CAD build for the part. Positions are in the model's coordinates, mm. A direction names the side the tool comes from. Round coordinates to 2 decimals unless told otherwise and drop trailing zeros. Write each loop counter-clockwise with the first axis right and the second up, starting at its lowest first coordinate (ties: lowest second). Pieces come first, ordered by that corner, then holes. Notation, with made-up numbers: (-4.5, 54.25) - (43.5, 54.25) arc R16 ccw to (43.5, 62.25) - close; hole circle Ø7 at (55.25, -33). An arc over 180 degrees is marked (long way). Answer in a Markdown table with one row per item.
Autodesk Inventor part; units mm, degrees
ref_plane "YZ Plane" through (0, 0, 0) normal (1, 0, 0) x (0, 1, 0)
ref_plane "XZ Plane" through (0, 0, 0) normal (0, 1, 0) x (-1, 0, 0)
ref_plane "XY Plane" through (0, 0, 0) normal (0, 0, 1) x (1, 0, 0)
sketch "Sketch1" plane through (0, 0, 0) normal (1, 0, 0) x (0, 1, 0)
  line L0 (-1.25, 6.25) -> (1.25, 6.25)
  arc A0 (1.25, -6.25) -> (1.25, 6.25) centre (1.25, 0) ccw
  line L1 (1.25, -6.25) -> (-1.25, -6.25)
  arc A1 (-1.25, 6.25) -> (-1.25, -6.25) centre (-1.25, 0) ccw
  circle A2 centre (0, -10) radius 1.6
  circle A3 centre (0, 10) radius 1.6
  circle A4 centre (8.25, 44.75) radius 1.6
  circle A5 centre (8.25, 65.25) radius 1.6
  line L2 (-1.25, 91.25) -> (1.25, 91.25)
  arc A6 (1.25, 78.75) -> (1.25, 91.25) centre (1.25, 85) ccw
  line L3 (1.25, 78.75) -> (-1.25, 78.75)
  arc A7 (-1.25, 91.25) -> (-1.25, 78.75) centre (-1.25, 85) ccw
  circle A8 centre (0, 75) radius 1.6
  circle A9 centre (0, 95) radius 1.6
  line L4 (-1.25, -91.25) -> (1.25, -91.25)
  arc A10 (1.25, -91.25) -> (1.25, -78.75) centre (1.25, -85) ccw
  line L5 (1.25, -78.75) -> (-1.25, -78.75)
  arc A11 (-1.25, -78.75) -> (-1.25, -91.25) centre (-1.25, -85) ccw
  circle A12 centre (0, -75) radius 1.6
  circle A13 centre (0, -95) radius 1.6
  circle A14 centre (-0.972, 44.75) radius 1.6
  circle A15 centre (-0.972, 65.25) radius 1.6
  circle A16 centre (8.25, -44.75) radius 1.6
  circle A17 centre (8.25, -65.25) radius 1.6
  circle A18 centre (-0.972, -44.75) radius 1.6
  circle A19 centre (-0.972, -65.25) radius 1.6
  arc A20 (12, 88) -> (-12, 88) centre (0, 88) ccw
  line L6 (12, 88) -> (12, -88)
  arc A21 (-12, -88) -> (12, -88) centre (0, -88) ccw
  line L7 (-12, -88) -> (-12, 88)
  point P0 (0, 0)
  point P1 (0, 0)
  point P2 (-12, -88)
  point P3 (12, 88)
  point P4 (-12, 88)
  point P5 (1.25, -78.75)
  point P6 (1.25, 78.75)
  point P7 (-1.25, 78.75)
  point P8 (1.25, -6.25)
  point P9 (-1.25, -6.25)
  dimension "d2" = 3.2
  dimension "d3" = 3.2
  dimension "d4" = 3.2
  dimension "d5" = 3.2
  dimension "d6" = 9.222
  dimension "d7" = 9.222
  dimension "d8" = 9.222
  dimension "d9" = 3.2
  dimension "d10" = 3.2
  dimension "d11" = 3.2
  dimension "d12" = 3.2
  dimension "d15" = 3.2
  dimension "d16" = 3.2
  dimension "d17" = 3.2
  dimension "d18" = 3.2
  dimension "d19" = 3.2
  dimension "d20" = 3.2
extrude "Extrusion1" add sketch "Sketch1" along normal blind 1
equation "\"d2\" = d5"
equation "\"d3\" = d5"
equation "\"d4\" = d5"
equation "\"d7\" = d6"
equation "\"d8\" = d6"
equation "\"d9\" = d5"
equation "\"d10\" = d5"
equation "\"d11\" = d5"
equation "\"d12\" = d5"
equation "\"d15\" = d5"
equation "\"d16\" = d5"
equation "\"d17\" = d5"
equation "\"d18\" = d5"
equation "\"d19\" = d5"
equation "\"d20\" = d5"
properties part number "Leg_Loadpipe_Plate_Outer" material "CFRP"
Q1. Saw through at A-A on z = -85. List the corners of the cut face in (x, y).
Computed:
| item | result |
|---|---|
| outline | (0, -12) - (1, -12) - (1, -7.5) - (0, -7.5) - close; (0, 7.5) - (1, 7.5) - (1, 12) - (0, 12) - close |
Q2. Saw through at C-C on y = 3.25. List the corners of the cut face in (x, z).
Computed:
| item | result |
|---|---|
| outline | (0, -99.55) - (1, -99.55) - (1, -90.92) - (0, -90.92) - close; (0, -79.08) - (1, -79.08) - (1, -5.92) - (0, -5.92) - close; (0, 5.92) - (1, 5.92) - (1, 79.08) - (0, 79.08) - close; (0, 90.92) - (1, 90.92) - (1, 99.55) - (0, 99.55) - close |
Q3. Saw through at B-B on x = 0.35. Count the separate pieces of the cut face and the enclosed holes in it, then the cut area to 3 significant figures.
Computed:
| item | result |
|---|---|
| separate pieces | 1 |
| enclosed holes | 17 |
| area | 4,100 mm2 |
Q4. Flat gauge pin, fed straight in: pin 1 (10 mm diameter, centred on y = -4.5, z = -49, fed in from -X). Where does the tip first touch, or does it go through?
Computed:
| item | result |
|---|---|
| pin 1 | stops at x = 0 |
Q5. Saw through at D-D on z = -3. List the corners of the cut face in (x, y).
Computed:
| item | result |
|---|---|
| outline | (0, -12) - (1, -12) - (1, -6.73) - (0, -6.73) - close; (0, 6.73) - (1, 6.73) - (1, 12) - (0, 12) - close |
Q6. 3-axis set-ups, long thin cutter, end or side, ignore diameter. For faces 1 (the flat face through (0, -8, 1)), 2 (the cylindrical face through (0.5, -7.5, -0.1)): which of +Z, -Z, +X, -X, +Y, -Y reach the whole face in a straight line?
Computed:
| item | result |
|---|---|
| face 1 | +Z, -Z, -X, +Y, -Y |
| face 2 | +X, -X |
Q7. Drill centre lines: line 1 (Y direction, x = 0.5, z = -65); line 2 (Z direction, x = 0.2, y = 5.5); line 3 (Y direction, x = 0.7, z = -75). Where is each one in solid material? Low to high.
Computed:
| item | result |
|---|---|
| line 1 | y = -12 to -2.55, 0.61 to 6.67, 9.83 to 12 |
| line 2 | z = -98.67 to -89.58, -80.42 to -4.58, 4.58 to 80.42, 89.58 to 98.67 |
| line 3 | y = -12 to -1.6, 1.6 to 12 |
